Autodesk Inventor part; units mm, degrees
ref_plane "YZ Plane" through (0, 0, 0) normal (1, 0, 0) x (0, 1, 0)
ref_plane "XZ Plane" through (0, 0, 0) normal (0, 1, 0) x (-1, 0, 0)
ref_plane "XY Plane" through (0, 0, 0) normal (0, 0, 1) x (1, 0, 0)
sketch "Esquisse1" plane through (0, 0, 0) normal (1, 0, 0) x (0, 1, 0)
  line L0 (0, 0) -> (25, 0)
  line L1 (25, 0) -> (25, -7.347)
  line L2 (25, -7.347) -> (0, -7.347)
  line L3 (0, -7.347) -> (0, 0)
  dimension "d0" = 25
  dimension "d1" = 7.347
extrude "Extrusion1" add sketch "Esquisse1" along normal blind 20
sketch "Esquisse3" plane through (20, 0, 0) normal (1, 0, 0) x (0, 0, -1)
  line L0 (0, 0) -> (7.347, 0)
  line L1 (0, 0) -> (3.5, 0)
  line L2 (3.5, 0) -> (3.5, 4)
  line L3 (7.347, 25) -> (0, 25)
  line L4 (0, 25) -> (3.5, 25)
  line L5 (3.5, 25) -> (3.5, 21)
  dimension "d7" = 3.5
  dimension "d8" = 4
  dimension "d9" = 3.5
  dimension "d10" = 4
  dimension "d11" = 90
hole "Perçage1" at (20, 4, -3.5) at (20, 21, -3.5) direction (-1, 0, 0) diameter 1.6 end through all
sketch "Esquisse4" plane through (0, 0, 0) normal (0, 0, 1) x (1, 0, 0)
  line L0 (0, 0) -> (20, 0)
  line L1 (0, 0) -> (14.4338, 25)
  line L2 (0, 25) -> (20, 25)
  line L3 (0, 0) -> (28.8675, 0) construction
  line L4 (0, 25) -> (20, 25)
  line L5 (20, 25) -> (20, 0)
  point P0 (10, 17.3205)
  dimension "d19" = 60
extrude "Extrusion3" cut sketch "Esquisse4" against normal blind 10
properties part number "face 30°"
The listing builds one solid part. Answer for the finished solid, in the listing's coordinates (mm). Coordinates: 2 decimals unless noted, no trailing zeros. Write each loop counter-clockwise with the first axis right and the second up, starting at its lowest first coordinate (ties: lowest second). Pieces come first, ordered by that corner, then holes. Notation, with made-up numbers: M 1,7 L 60,7 A21 ccw 60,17 Z; hole C 0,20 d11. An arc over 180 degrees is marked long. Use a Markdown table: item, result. Add a question column.
1. Section D-D (z = -6) is taken. Give the vertices of the cut face in (x, y), plus the area to 3 significant figures.
2. Section B-B (y = 4) is taken. Give the vertices of the cut face in (x, z).
3. For a pull along Z with two mould halves and no side action, classify faces 1 (the flat face through (4, 18, 0)), 2 (the flat face through (7.1, 12.3, -3.6)), 3 (the cylindrical face through (1.06, 4.78, -3.33)) as +Z half, -Z half, draft (parallel to the pull), parting line (faces both ways), or undercut.
4. Straight lines are drawn through the part: line 1 along Z through (x, y) = (1.65, 4); line 2 along Y through (x, z) = (1.25, -3.5); line 3 along Y through (x, z) = (1, -3.5). For each, find the intervals that lie inside material, in ascending order. Write a range as [from, to].
5. Section C-C (x = 9.5) is taken. Give the vertices of the cut face in (y, z), plus the area to 3 significant figures.
6. Given P1, Ø3, axis at x = 4, z = -4, coming from the -Y side; P2, Ø1.5, axis at y = 13, z = -6.5, coming from the +X side; P3, Ø8, axis at x = 4, y = 21, coming from the +Z side; P4, Ø2, axis at y = 4, z = -3.5, coming from the +X side, each flat-ended and moving along its own axis, determine where each tip first touches the part or whether it passes through.
7. Section A-A (z = -3.5) is taken. Give the vertices of the cut face in (x, y).
Data:
| question | item | result |
|---|---|---|
| 1 | outline | M 0,0 L 14.43,25 L 0,25 Z |
| 1 | area | 180 mm2 |
| 2 | outline | M 0,-7.35 L 2.31,-7.35 L 2.31,-4.3 L 0,-4.3 Z; M 0,-2.7 L 2.31,-2.7 L 2.31,0 L 0,0 Z |
| 3 | face 1 | +Z half |
| 3 | face 2 | draft |
| 3 | face 3 | undercut |
| 4 | line 1 | z = [-7.35, -4.3], [-2.7, 0] |
| 4 | line 2 | y = [2.17, 3.2], [4.8, 20.2], [21.8, 25] |
| 4 | line 3 | y = [1.73, 3.2], [4.8, 20.2], [21.8, 25] |
| 5 | outline | M 16.45,-7.35 L 25,-7.35 L 25,0 L 16.45,0 Z; hole C 21,-3.5 d1.6 |
| 5 | area | 60.8 mm2 |
| 6 | P1 | stops at y = 4.36 |
| 6 | P2 | stops at x = 7.94 |
| 6 | P3 | stops at z = 0 |
| 6 | P4 | stops at x = 2.89 |
| 7 | outline | M 0,0 L 1.85,3.2 L 0,3.2 Z; M 0,4.8 L 2.77,4.8 L 11.66,20.2 L 0,20.2 Z; M 0,21.8 L 12.59,21.8 L 14.43,25 L 0,25 Z |
